Geometry: final body of the model. Coordinates: model frame, mm. Round coordinates to 2 decimals unless told otherwise and drop trailing zeros. Write each loop counter-clockwise with the first axis right and the second up, starting at its lowest first coordinate (ties: lowest second). Pieces come first, ordered by that corner, then holes. Notation, with made-up numbers: (85, 63) - (101, 63) arc R12 cw to (101, 83) - close; hole circle Ø10 at (17, 11). An arc over 180 degrees is marked (long way). Write each question's results on one line, items separated by ' | '.
from build123d import *

# Parameters (mm, degrees)
ESQUISSE1_R      = 0.75
EXTRUSION1_DEPTH = 0.7


with BuildPart() as part:
    # Esquisse1 → Extrusion1 (new body)
    with BuildSketch(Plane.XY):
        with BuildLine():
            Line((-6.5, -1), (-6.5, 6.144102864))
            ThreePointArc((-6.5, 6.144102864), (-6.485251672, 6.2194807), (-6.443181818, 6.283741565))
            ThreePointArc((-6.443181818, 6.283741565), (-4.741623269, 7.649641088), (-2.761363636, 8.565913312))
            ThreePointArc((-2.761363636, 8.565913312), (-2.582256056, 8.53722713), (-2.5, 8.375559683))
            Line((-2.5, 8.375559683), (-2.5, 5.133225107))
            ThreePointArc((-2.5, 5.133225107), (-2.528797357, 5.029834318), (-2.606896552, 4.956217345))
            ThreePointArc((-2.606896552, 4.956217345), (0, -5.6), (2.606896552, 4.956217345))
            ThreePointArc((2.606896552, 4.956217345), (2.528797357, 5.029834318), (2.5, 5.133225107))
            Line((2.5, 5.133225107), (2.5, 8.375559683))
            ThreePointArc((2.5, 8.375559683), (2.582256056, 8.53722713), (2.761363636, 8.565913312))
            ThreePointArc((2.761363636, 8.565913312), (4.741623269, 7.649641088), (6.443181818, 6.283741565))
            ThreePointArc((6.443181818, 6.283741565), (6.485251672, 6.2194807), (6.5, 6.144102864))
            Line((6.5, 6.144102864), (6.5, -1))
            ThreePointArc((6.5, -1), (0, -7.5), (-6.5, -1))
        make_face()
        with Locations((-4.5, 5.75)):
            Circle(ESQUISSE1_R, mode=Mode.SUBTRACT)
        with Locations(Location((4.5, 5.75, 0), (0, 0, 180))):
            Circle(ESQUISSE1_R, mode=Mode.SUBTRACT)
    extrude(amount=EXTRUSION1_DEPTH)


solid = part.part
Q1. Mould query, pull axis Y, two halves, no side actions, for faces 1 (the cylindrical face through (-5.25, 5.78, 0.35)), 2 (the cylindrical face through (-0.208, -5.596, 0.345)), 3 (the cylindrical face through (4.716, 7.666, 0.345)), 4 (the cylindrical face through (0.1, -7.5, 0.3)). Classes: pulls with the +Y half, pulls with the -Y half, needs draft (parallel to the pull), parting line crosses it, or undercut.
Answer block:
face 1: undercut | face 2: undercut | face 3: pulls with the +Y half | face 4: pulls with the -Y half
Q2. Section query A-A, the plane y = 5.75. Return loops of the section in (x, z), plus the area to 3 significant figures.
Answer block:
outline: (-6.5, 0) - (-5.25, 0) - (-5.25, 0.7) - (-6.5, 0.7) - close; (-3.75, 0) - (-2.5, 0) - (-2.5, 0.7) - (-3.75, 0.7) - close; (2.5, 0) - (3.75, 0) - (3.75, 0.7) - (2.5, 0.7) - close; (5.25, 0) - (6.5, 0) - (6.5, 0.7) - (5.25, 0.7) - close | area: 3.50 mm2
Q3. Section query B-B, the plane y = 0. Return loops of the section in (x, z).
Answer block:
outline: (-6.5, 0) - (-5.6, 0) - (-5.6, 0.7) - (-6.5, 0.7) - close; (5.6, 0) - (6.5, 0) - (6.5, 0.7) - (5.6, 0.7) - close
Q4. Ray query, line 1 along X through (y, z) = (0, 0.3); line 2 along Y through (x, z) = (-4.5, 0.2); line 3 along X through (y, z) = (5.5, 0.3). Return the intervals inside material, ascending.
Answer block:
line 1: -6.5 to -5.6, 5.6 to 6.5 | line 2: -5.69 to -3.33, 3.33 to 5, 6.5 to 7.79 | line 3: -6.5 to -5.21, -3.79 to -2.5, 2.5 to 3.79, 5.21 to 6.5
Q5. Section query C-C, the plane x = 3. Return loops of the section in (y, z).
Answer block:
outline: (-6.77, 0) - (-4.73, 0) - (-4.73, 0.7) - (-6.77, 0.7) - close; (4.73, 0) - (8.49, 0) - (8.49, 0.7) - (4.73, 0.7) - close
Q6. Section query D-D, the plane z = 0.15. Return loops of the section in (x, y).
Answer block:
outline: (-6.5, -1) arc R6.5 ccw to (6.5, -1) - (6.5, 6.14) arc R0.2 ccw to (6.44, 6.28) arc R9 ccw to (2.76, 8.57) arc R0.2 ccw to (2.5, 8.38) - (2.5, 5.13) arc R0.2 ccw to (2.61, 4.96) arc R5.6 cw (long way) to (-2.61, 4.96) arc R0.2 ccw to (-2.5, 5.13) - (-2.5, 8.38) arc R0.2 ccw to (-2.76, 8.57) arc R9 ccw to (-6.44, 6.28) arc R0.2 ccw to (-6.5, 6.14) - close; hole circle Ø1.5 at (-4.5, 5.75); hole circle Ø1.5 at (4.5, 5.75)
